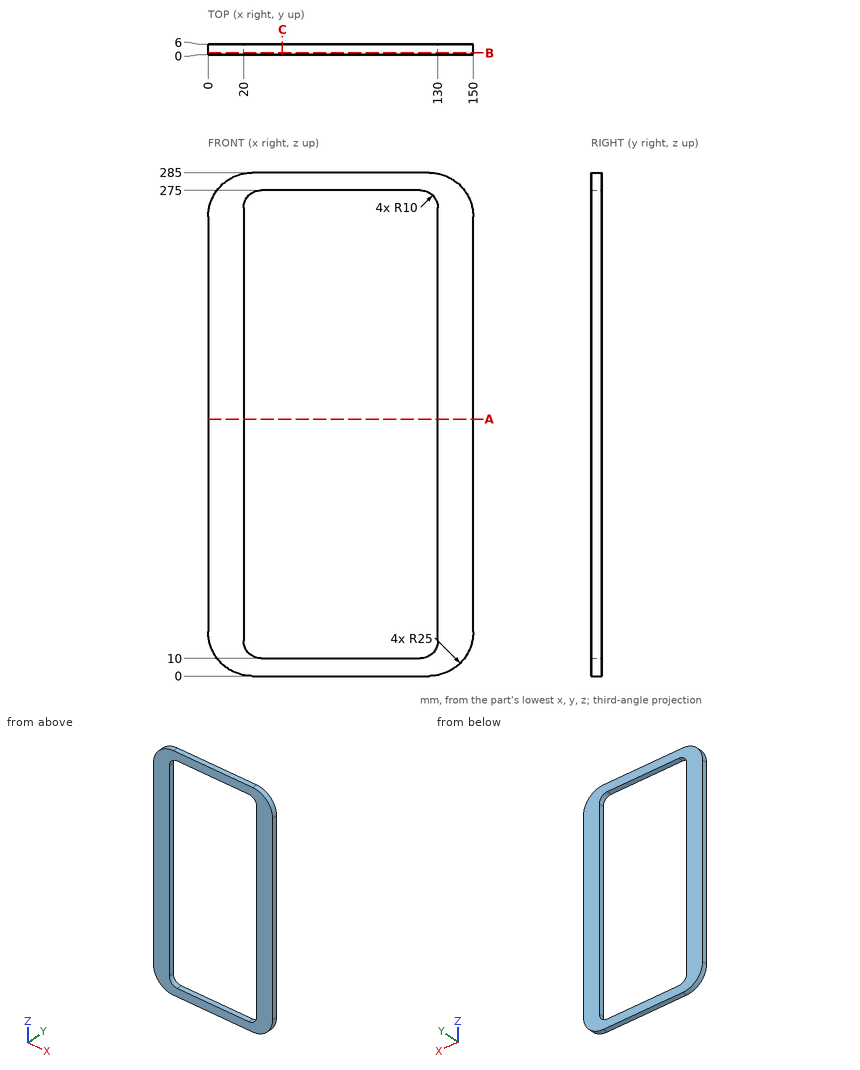
Design review of the part shown in the three views and the two pictorial views. Dimensions are in mm from the part's minimum x, y and z. Give positions to 0.01 mm unless a question says otherwise; leave off trailing zeros. Write each loop counter-clockwise with the first axis right and the second up, starting at its lowest first coordinate (ties: lowest second). Pieces come first, ordered by that corner, then holes.
Item 1: Take a section at C-C (x = 42). Give the boundary of the cut face in (y, z).
Item 2: Take a section at B-B (y = 1). Give the boundary of the cut face in (x, z).
Item 3: Take a section at A-A (z = 145.5). Give the boundary of the cut face in (x, y).
Item 4: Insertion check: P1, Ø3, axis at x = 132, y = 0.5, coming from the +Z side. The pin has a flat end and moves straight along its axis. Give the tip position at first contact, or say it passes through.
Item 5: Wall thickness on probe 1 along X at (y, z) = (3.1, 179.5); probe 2 along Z at (x, y) = (95, 3.7); probe 3 along Z at (x, y) = (17, 0.75): over which ranges is each line inside the solid? List them lowest first.
Established:
1. outline: (0, 0) - (6, 0) - (6, 10) - (0, 10) - close; (0, 275) - (6, 275) - (6, 285) - (0, 285) - close
2. outline: (0, 25) arc R25 ccw to (25, 0) - (125, 0) arc R25 ccw to (150, 25) - (150, 260) arc R25 ccw to (125, 285) - (25, 285) arc R25 ccw to (0, 260) - close; hole (20, 20) arc R10 ccw to (30, 10) - (120, 10) arc R10 ccw to (130, 20) - (130, 265) arc R10 ccw to (120, 275) - (30, 275) arc R10 ccw to (20, 265) - close
3. outline: (0, 0) - (20, 0) - (20, 6) - (0, 6) - close; (130, 0) - (150, 0) - (150, 6) - (130, 6) - close
4. P1: stops at z = 284.39
5. probe 1: x = 0 to 20, 130 to 150
5. probe 2: z = 0 to 10, 275 to 285
5. probe 3: z = 1.31 to 283.69
